Work out the finished part from the listing and answer in its coordinate system (mm). Face numbers are marked on the shaded views. A direction names the side the tool comes from. Give positions to 0.01 mm unless a question says otherwise; leave off trailing zeros. Order: outer loops, then holes, each group sorted by start corner. A loop starts at its lowest first (then second) coordinate and runs counter-clockwise, first axis right, second up. Notation, with made-up numbers: (-12, 31) -> (26, 31) arc R28 cw to (26, 62) -> close; hole circle Ø10 at (-12, 58.25). An arc over 180 degrees is marked (long way). Answer as CSV lines item,"result". Start each with the question number.
1. A cutting plane is placed at C-C (y = 2.5). Give the vertices of the cut face in (x, z).
2. Find the intervals of material crossed by L1, parallel to X at y = 1.2, z = -12.7; L2, parallel to Z at x = -12.7, y = 2.4; L3, parallel to Z at x = -12.7, y = 3.25, in increasing order.
3. For the marked faces 1, 2 and 3, determine the directions among +Z, -Z, +X, -X, +Y, -Y from which every point of the face is accessible in a straight line to the end or side of a thin tool.
4. Flat-ended cylindrical pins translate along their axes: pin 1 (2.5 mm diameter, centred on x = 2, y = 5.5, fed in from +Z); pin 2 (6.5 mm diameter, centred on x = -9, z = 11, fed in from +Y) (3 decimals); pin 3 (3.5 mm diameter, centred on x = 9, y = 5, fed in from -Z). Find the tip coordinate at first contact, or state that the pin passes through.
5. A cutting plane is placed at A-A (z = -12.7). Give the vertices of the cut face in (x, y) (3 decimals), then the cut area to 3 significant figures.
6. A cutting plane is placed at D-D (x = -0.5). Give the vertices of the cut face in (y, z) (3 decimals).
7. A cutting plane is placed at B-B (x = 12.7). Give the vertices of the cut face in (y, z) (3 decimals).
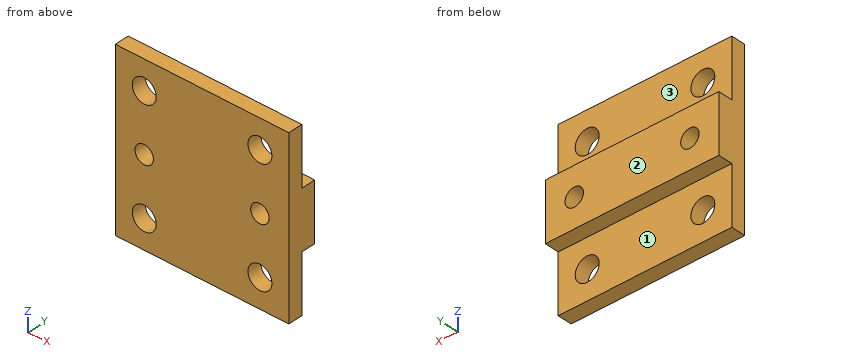
from build123d import *

# Parameters (mm, degrees)
SKETCH1_W           = 38.1
SKETCH1_H           = 38.1
SKETCH1_R           = 2.0193
SKETCH1_R_2         = 2.6289
BOSS_EXTRUDE4_DEPTH = 6.35
SKETCH12_W          = 38.1
SKETCH12_H          = 12.7
CUT_EXTRUDE7_DEPTH  = 3.175


with BuildPart() as part:
    # Sketch1 → Boss-Extrude4 (new body)
    with BuildSketch(Plane(origin=(0, 0, 0), x_dir=(1, 0, 0), z_dir=(0, 1, 0))):
        Rectangle(SKETCH1_W, SKETCH1_H)
        with Locations((-12.7, 0)):
            Circle(SKETCH1_R, mode=Mode.SUBTRACT)
        with Locations((12.7, 0)):
            Circle(SKETCH1_R, mode=Mode.SUBTRACT)
        with Locations((-12.7, 12.7)):
            Circle(SKETCH1_R_2, mode=Mode.SUBTRACT)
        with Locations((12.7, 12.7)):
            Circle(SKETCH1_R_2, mode=Mode.SUBTRACT)
        with Locations((12.7, -12.7)):
            Circle(SKETCH1_R_2, mode=Mode.SUBTRACT)
        with Locations((-12.7, -12.7)):
            Circle(SKETCH1_R_2, mode=Mode.SUBTRACT)
    extrude(amount=BOSS_EXTRUDE4_DEPTH)

    # Sketch12 → Cut-Extrude7 (cut)
    with BuildSketch(Plane(origin=(0, 6.35, 0), x_dir=(1, 0, 0), z_dir=(0, 1, 0))):
        with Locations((0, 12.7)):
            Rectangle(SKETCH12_W, SKETCH12_H)
        with Locations((0, -12.7)):
            Rectangle(SKETCH12_W, SKETCH12_H)
    extrude(amount=-CUT_EXTRUDE7_DEPTH, mode=Mode.SUBTRACT)


solid = part.part
Answer sheet:
1,outline,"(-19.05, -19.05) -> (19.05, -19.05) -> (19.05, 19.05) -> (-19.05, 19.05) -> close; hole circle Ø5.26 at (-12.7, -12.7); hole circle Ø5.26 at (-12.7, 12.7); hole circle Ø4.04 at (-12.7, 0); hole circle Ø5.26 at (12.7, -12.7); hole circle Ø5.26 at (12.7, 12.7); hole circle Ø4.04 at (12.7, 0)"
2,L1,"x = -19.05 to -15.33, -10.07 to 10.07, 15.33 to 19.05"
2,L2,"z = -19.05 to -15.33, -10.07 to -2.02, 2.02 to 10.07, 15.33 to 19.05"
2,L3,"z = -6.35 to -2.02, 2.02 to 6.35"
3,face 1,"-Z, +X, -X, +Y"
3,face 2,"+Z, -Z, +X, -X, +Y"
3,face 3,"+Z, +X, -X, +Y"
4,pin 1,"stops at z = 6.35"
4,pin 2,"stops at y = 3.175"
4,pin 3,"stops at z = -6.35"
5,outline,"(-19.05, 0) -> (-15.329, 0) -> (-15.329, 3.175) -> (-19.05, 3.175) -> close; (-10.071, 0) -> (10.071, 0) -> (10.071, 3.175) -> (-10.071, 3.175) -> close; (15.329, 0) -> (19.05, 0) -> (19.05, 3.175) -> (15.329, 3.175) -> close"
5,area,"87.6 mm^2"
6,outline,"(0, -19.05) -> (3.175, -19.05) -> (3.175, -6.35) -> (6.35, -6.35) -> (6.35, 6.35) -> (3.175, 6.35) -> (3.175, 19.05) -> (0, 19.05) -> close"
7,outline,"(0, -19.05) -> (3.175, -19.05) -> (3.175, -15.329) -> (0, -15.329) -> close; (0, -10.071) -> (3.175, -10.071) -> (3.175, -6.35) -> (6.35, -6.35) -> (6.35, -2.019) -> (0, -2.019) -> close; (0, 2.019) -> (6.35, 2.019) -> (6.35, 6.35) -> (3.175, 6.35) -> (3.175, 10.071) -> (0, 10.071) -> close; (0, 15.329) -> (3.175, 15.329) -> (3.175, 19.05) -> (0, 19.05) -> close"
